Geometry: final body of the model. Coordinates: model frame, mm. A direction names the side the tool comes from. Give positions to 0.01 mm unless a question says otherwise; leave off trailing zeros. Write each loop counter-clockwise with the first axis right and the second up, starting at its lowest first coordinate (ties: lowest second). Pieces come first, ordered by that corner, then holes. Notation, with made-up numbers: M -13.5,85 L 0.5,85 A25 cw 0.5,103 Z; hole C -0.75,84.25 d5. An arc over 180 degrees is marked long. Use a Markdown table: item, result. Add a question column.
(1) Pin query (flat end, axial travel): pin 1 Ø1.7 at (x, z) = (-23, 13) entering from +Y; pin 2 Ø5 at (y, z) = (3, 16) entering from -X; pin 3 Ø4 at (x, z) = (0, -27) entering from +Y. Return the tip coordinate at first contact, or that it passes through.
(2) Draft query along Z for faces 1 (the flat face through (16, 43, 17)), 2 (the flat face through (-4.5, 2, 15)), 3 (the cylindrical face through (16.87, 12.29, 5.85)). Return one class per face: released by +Z, released by -Z, zero draft, split by the parting line, or undercut.
(3) Cut plane B-B (y = 35.15). Output: boundary loops of the cut face in (x, z).
(4) Cut plane D-D (x = -16.9). State how many separate pieces and enclosed holes the cut face has, plus the area to 3 significant figures.
(5) Cut plane A-A (y = 49.5). Output: boundary loops of the cut face in (x, z), plus the area to 3 significant figures.
(6) Cut plane C-C (z = 0). Output: boundary loops of the cut face in (x, y).
(7) Material intervals for L1, parallel to Z at x = 17, y = 11; L2, parallel to X at y = 71.5, z = -4.5; L3, parallel to Y at x = 23, z = -7, sorted ascending.
(8) Reachability of faces 4 (the flat face through (0, -2.3, -5)), 5 (the flat face through (9, -12, -22.1)), 6 (the flat face through (19.4, 41, 0)), 7 (the flat face through (-19.4, 41, 0)), 8 (the cylindrical face through (15.68, 78.07, -14.77)) from +Z, -Z, +X, -X, +Y, -Y: full face, straight path, thin tool, end or side. Return the list, or none.
```python
from build123d import *

# Parameters (mm, degrees)
CROQUIS2_R              = 33
SALIENTE_EXTRUIR1_DEPTH = 1
SALIENTE_EXTRUIR2_START = 6.3
CROQUIS3_R              = 33
CROQUIS3_R_2            = 27.85
SALIENTE_EXTRUIR2_DEPTH = 6.3
CROQUIS4_W              = 5
CROQUIS4_H              = 34
SALIENTE_EXTRUIR3_DEPTH = 82
CROQUIS5_W              = 28.8
CROQUIS5_H              = 34
SALIENTE_EXTRUIR4_DEPTH = 3.3
CROQUIS6_R              = 1.5
CORTAR_EXTRUIR1_DEPTH   = 5
REDONDEO2_R             = 2.8
CROQUIS7_R              = 1.25
CORTAR_EXTRUIR2_DEPTH   = 10
CROQUIS9_R              = 30
CROQUIS9_R_2            = 23.65
SALIENTE_EXTRUIR5_DEPTH = 12
CROQUIS10_R             = 23.65
SALIENTE_EXTRUIR6_DEPTH = 6.3
CROQUIS12_R             = 1.65
CORTAR_EXTRUIR4_DEPTH   = 4
CROQUIS13_R             = 1.68
CORTAR_EXTRUIR5_DEPTH   = 5
CORTAR_EXTRUIR9_REACH   = 102.76
CROQUIS14_R             = 4.5
CROQUIS16_W             = 28.8
CROQUIS16_H             = 34
CORTAR_EXTRUIR11_DEPTH  = 0.4
CORTAR_EXTRUIR12_START  = -2.9
CORTAR_EXTRUIR12_DEPTH  = 2.9
CORTAR_EXTRUIR13_REACH  = 105.556
CROQUIS18_R             = 1.15


with BuildPart() as part:
    # Croquis2 → Saliente-Extruir1 (new body)
    with BuildSketch(Plane(origin=(0, 0, 0), x_dir=(1, 0, 0), z_dir=(0, 1, 0))):
        with Locations(Location((0, 0, 0), (0, 0, 270))):
            Circle(CROQUIS2_R)
    extrude(amount=SALIENTE_EXTRUIR1_DEPTH)

    # Croquis3 → Saliente-Extruir2 (add)
    with BuildSketch(Plane.XZ.offset(SALIENTE_EXTRUIR2_START)):
        with Locations(Location((0, 0, 0), (0, 0, 270))):
            Circle(CROQUIS3_R)
        with Locations(Location((0, 0, 0), (0, 0, 270))):
            Circle(CROQUIS3_R_2, mode=Mode.SUBTRACT)
    extrude(amount=-SALIENTE_EXTRUIR2_DEPTH)

    # Croquis4 → Saliente-Extruir3 (add)
    with BuildSketch(Plane(origin=(0, 1, 0), x_dir=(1, 0, 0), z_dir=(0, 1, 0))):
        with Locations((-16.9, 0)):
            Rectangle(CROQUIS4_W, CROQUIS4_H)
        with Locations((16.9, 0)):
            Rectangle(CROQUIS4_W, CROQUIS4_H)
    extrude(amount=SALIENTE_EXTRUIR3_DEPTH)

    # Croquis5 → Saliente-Extruir4 (add)
    with BuildSketch(Plane(origin=(0, 1, 0), x_dir=(1, 0, 0), z_dir=(0, 1, 0))):
        Rectangle(CROQUIS5_W, CROQUIS5_H)
    extrude(amount=SALIENTE_EXTRUIR4_DEPTH)

    # Croquis6 → Cortar-Extruir1 (cut)
    with BuildSketch(Plane(origin=(0, 1, 0), x_dir=(1, 0, 0), z_dir=(0, 1, 0))):
        with Locations(Location((23.382685902, 13.5, 0), (0, 0, 270))):
            Circle(CROQUIS6_R)
        with Locations(Location((0, 27, 0), (0, 0, 270))):
            Circle(CROQUIS6_R)
        with Locations(Location((23.382685902, -13.5, 0), (0, 0, 270))):
            Circle(CROQUIS6_R)
        with Locations(Location((0, -27, 0), (0, 0, 270))):
            Circle(CROQUIS6_R)
        with Locations(Location((-23.382685902, -13.5, 0), (0, 0, 270))):
            Circle(CROQUIS6_R)
        with Locations(Location((-23.382685902, 13.5, 0), (0, 0, 270))):
            Circle(CROQUIS6_R)
    extrude(amount=-CORTAR_EXTRUIR1_DEPTH, mode=Mode.SUBTRACT)

    # Redondeo2
    redondeo2_edges = [part.edges().sort_by_distance(p)[0] for p in [
        (0, 1, 17),
        (0, 1, -17),
    ]]
    fillet(redondeo2_edges, radius=REDONDEO2_R)

    # Croquis7 → Cortar-Extruir2 (cut)
    with BuildSketch(Plane(origin=(0, 83, 0), x_dir=(1, 0, 0), z_dir=(0, 1, 0))):
        with Locations(Location((16.9, 14.5, 0), (0, 0, 270))):
            Circle(CROQUIS7_R)
        with Locations(Location((-16.9, 14.5, 0), (0, 0, 270))):
            Circle(CROQUIS7_R)
        with Locations(Location((-16.9, -14.5, 0), (0, 0, 270))):
            Circle(CROQUIS7_R)
        with Locations(Location((16.9, -14.5, 0), (0, 0, 270))):
            Circle(CROQUIS7_R)
    extrude(amount=-CORTAR_EXTRUIR2_DEPTH, mode=Mode.SUBTRACT)

    # Croquis9 → Saliente-Extruir5 (add)
    with BuildSketch(Plane.XZ):
        with Locations(Location((0, 0, 0), (0, 0, 270))):
            Circle(CROQUIS9_R)
        with Locations(Location((0, 0, 0), (0, 0, 270))):
            Circle(CROQUIS9_R_2, mode=Mode.SUBTRACT)
    extrude(amount=SALIENTE_EXTRUIR5_DEPTH)

    # Croquis10 → Saliente-Extruir6 (add)
    with BuildSketch(Plane.XZ):
        with Locations(Location((0, 0, 0), (0, 0, 270))):
            Circle(CROQUIS10_R)
    extrude(amount=SALIENTE_EXTRUIR6_DEPTH)

    # Croquis11 → Revolución1 (revolve)
    with BuildSketch(Plane(origin=(0, 0, 0), x_dir=(0, 0, -1), z_dir=(1, 0, 0))):
        Polygon((33, -6.3), (30, -6.3), (30, -12), align=None)
    revolve(axis=Axis((0, -12, 0), (0, 1, 0)))

    # Croquis12 → Cortar-Extruir4 (cut)
    with BuildSketch(Plane.XZ.offset(6.3)):
        with Locations(Location((-8.7777e-05, -5.499999999, 0), (0, 0, 270))):
            Circle(CROQUIS12_R)
        with Locations(Location((5.499999999, -8.7777e-05, 0), (0, 0, 270))):
            Circle(CROQUIS12_R)
        with Locations(Location((-5.499999999, 8.7777e-05, 0), (0, 0, 270))):
            Circle(CROQUIS12_R)
        with Locations(Location((8.7777e-05, 5.499999999, 0), (0, 0, 270))):
            Circle(CROQUIS12_R)
    extrude(amount=-CORTAR_EXTRUIR4_DEPTH, mode=Mode.SUBTRACT)

    # Croquis13 → Cortar-Extruir5 (cut)
    with BuildSketch(Plane(origin=(0, 1, 0), x_dir=(1, 0, 0), z_dir=(0, 1, 0))):
        with Locations(Location((-23.382685902, 13.5, 0), (0, 0, 270))):
            Circle(CROQUIS13_R)
        with Locations(Location((0, 27, 0), (0, 0, 270))):
            Circle(CROQUIS13_R)
        with Locations(Location((23.382685902, 13.5, 0), (0, 0, 270))):
            Circle(CROQUIS13_R)
        with Locations(Location((23.382685902, -13.5, 0), (0, 0, 270))):
            Circle(CROQUIS13_R)
        with Locations(Location((0, -27, 0), (0, 0, 270))):
            Circle(CROQUIS13_R)
        with Locations(Location((-23.382685902, -13.5, 0), (0, 0, 270))):
            Circle(CROQUIS13_R)
    extrude(amount=-CORTAR_EXTRUIR5_DEPTH, mode=Mode.SUBTRACT)

    # Croquis14 → Cortar-Extruir9 (cut, up to next)
    with BuildSketch(Plane.XZ.offset(6.3), mode=Mode.PRIVATE) as cortar_extruir9_sk1:
        with Locations(Location((0, 11.999999999, 0), (0, 0, 270))):
            Circle(CROQUIS14_R)
    cortar_extruir9_tool1 = extrude(cortar_extruir9_sk1.sketch, amount=-CORTAR_EXTRUIR9_REACH, mode=Mode.PRIVATE) & part.part
    add(cortar_extruir9_tool1.solids().sort_by_distance((0, -6.3, 12))[0], mode=Mode.SUBTRACT)

    # Croquis16 → Cortar-Extruir11 (cut)
    with BuildSketch(Plane(origin=(0, 4.3, 0), x_dir=(1, 0, 0), z_dir=(0, 1, 0))):
        Rectangle(CROQUIS16_W, CROQUIS16_H)
    extrude(amount=-CORTAR_EXTRUIR11_DEPTH, mode=Mode.SUBTRACT)

    # Croquis17 → Cortar-Extruir12 (cut)
    with BuildSketch(Plane(origin=(0, 3.9, 0), x_dir=(1, 0, 0), z_dir=(0, 1, 0)).offset(CORTAR_EXTRUIR12_START)):
        with BuildLine():
            Line((-4.5, -11.999999999), (-4.5, -19.8))
            Line((-4.5, -19.8), (4.5, -19.8))
            Line((4.5, -19.8), (4.5, -11.999999999))
            ThreePointArc((4.5, -11.999999999), (0, -16.499999999), (-4.5, -11.999999999))
        make_face()
    extrude(amount=CORTAR_EXTRUIR12_DEPTH, mode=Mode.SUBTRACT)

    # Cortar-Extruir13: up to this face of the body (flat: up to its plane)
    cortar_extruir13_end = Plane(part.part.faces().sort_by_distance((19.4, 41.951328943, 0))[0])
    # Croquis18 → Cortar-Extruir13 (cut, up to the picked face)
    with BuildSketch(Plane.ZY.offset(19.4), mode=Mode.PRIVATE) as cortar_extruir13_sk1:
        with Locations((6, 11.15)):
            Circle(CROQUIS18_R)
    cortar_extruir13_tool1 = split(extrude(cortar_extruir13_sk1.sketch, amount=-CORTAR_EXTRUIR13_REACH, mode=Mode.PRIVATE), bisect_by=cortar_extruir13_end, keep=Keep.BOTH, mode=Mode.PRIVATE)
    # Croquis18 → Cortar-Extruir13 (cut, up to the picked face)
    with BuildSketch(Plane.ZY.offset(19.4), mode=Mode.PRIVATE) as cortar_extruir13_sk2:
        with Locations((-6, 11.15)):
            Circle(CROQUIS18_R)
    cortar_extruir13_tool2 = split(extrude(cortar_extruir13_sk2.sketch, amount=-CORTAR_EXTRUIR13_REACH, mode=Mode.PRIVATE), bisect_by=cortar_extruir13_end, keep=Keep.BOTH, mode=Mode.PRIVATE)
    # Croquis18 → Cortar-Extruir13 (cut, up to the picked face)
    with BuildSketch(Plane.ZY.offset(19.4), mode=Mode.PRIVATE) as cortar_extruir13_sk3:
        with Locations((-6, 35.15)):
            Circle(CROQUIS18_R)
    cortar_extruir13_tool3 = split(extrude(cortar_extruir13_sk3.sketch, amount=-CORTAR_EXTRUIR13_REACH, mode=Mode.PRIVATE), bisect_by=cortar_extruir13_end, keep=Keep.BOTH, mode=Mode.PRIVATE)
    # Croquis18 → Cortar-Extruir13 (cut, up to the picked face)
    with BuildSketch(Plane.ZY.offset(19.4), mode=Mode.PRIVATE) as cortar_extruir13_sk4:
        with Locations((6, 35.15)):
            Circle(CROQUIS18_R)
    cortar_extruir13_tool4 = split(extrude(cortar_extruir13_sk4.sketch, amount=-CORTAR_EXTRUIR13_REACH, mode=Mode.PRIVATE), bisect_by=cortar_extruir13_end, keep=Keep.BOTH, mode=Mode.PRIVATE)
    add(cortar_extruir13_tool1.solids().sort_by(Axis((-19.4, 11.15, 6), (1, 0, 0)))[0], mode=Mode.SUBTRACT)
    add(cortar_extruir13_tool2.solids().sort_by(Axis((-19.4, 11.15, -6), (1, 0, 0)))[0], mode=Mode.SUBTRACT)
    add(cortar_extruir13_tool3.solids().sort_by(Axis((-19.4, 35.15, -6), (1, 0, 0)))[0], mode=Mode.SUBTRACT)
    add(cortar_extruir13_tool4.solids().sort_by(Axis((-19.4, 35.15, 6), (1, 0, 0)))[0], mode=Mode.SUBTRACT)


solid = part.part
```
Answer list:
| question | item | result |
|---|---|---|
| 1 | pin 1 | y = -4 |
| 1 | pin 2 | x = -29.64 |
| 1 | pin 3 | y = 1 |
| 2 | face 1 | released by +Z |
| 2 | face 2 | zero draft |
| 2 | face 3 | undercut |
| 3 | outline | M -19.4,-17 L -14.4,-17 L -14.4,-7.15 L -19.4,-7.15 Z; M -19.4,-4.85 L -14.4,-4.85 L -14.4,4.85 L -19.4,4.85 Z; M -19.4,7.15 L -14.4,7.15 L -14.4,17 L -19.4,17 Z; M 14.4,-17 L 19.4,-17 L 19.4,-7.15 L 14.4,-7.15 Z; M 14.4,-4.85 L 19.4,-4.85 L 19.4,4.85 L 14.4,4.85 Z; M 14.4,7.15 L 19.4,7.15 L 19.4,17 L 14.4,17 Z |
| 4 | separate pieces | 1 |
| 4 | enclosed holes | 4 |
| 4 | area | 3,250 mm² |
| 5 | outline | M -19.4,-17 L -14.4,-17 L -14.4,17 L -19.4,17 Z; M 14.4,-17 L 19.4,-17 L 19.4,17 L 14.4,17 Z |
| 5 | area | 340 mm² |
| 6 | outline | M -33,-6.3 L -30,-12 L -23.65,-12 L -23.65,-6.3 L -7.15,-6.3 L -7.15,-2.3 L -3.85,-2.3 L -3.85,-6.3 L 3.85,-6.3 L 3.85,-2.3 L 7.15,-2.3 L 7.15,-6.3 L 23.65,-6.3 L 23.65,-12 L 30,-12 L 33,-6.3 L 33,1 L 19.4,1 L 19.4,83 L 14.4,83 L 14.4,3.9 L -14.4,3.9 L -14.4,83 L -19.4,83 L -19.4,1 L -33,1 Z |
| 7 | L1 | -17 to -7.14, -4.86 to 4.86, 7.14 to 17 |
| 7 | L2 | -19.4 to -14.4, 14.4 to 19.4 |
| 7 | L3 | -12 to 1 |
| 8 | face 4 | -Y |
| 8 | face 5 | +Z, -Z, +X, -X, -Y |
| 8 | face 6 | +Z, -Z, +X, +Y |
| 8 | face 7 | +Z, -Z, -X, +Y |
| 8 | face 8 | +Y |
